The model under review builds one solid part; all positions refer to its coordinate system, in mm. A direction names the side the tool comes from. Give positions to 0.01 mm unless a question says otherwise; leave off trailing zeros. Loops run counter-clockwise (first coordinate to the right, second up) from the corner with the lowest first, then second, coordinate; pieces in that order, holes last. Notation, with made-up numbers: M 13,-29 L 63,-29 A28 ccw 63,-6 Z; hole C 12.25,41.25 d3. An arc over 180 degrees is marked long. Put each result on its own line as item: value. Start each with the question number.
from build123d import *

# Parameters (mm, degrees)
SKETCH1_W           = 30
SKETCH1_H           = 15
BOSS_EXTRUDE1_DEPTH = 3
SKETCH2_W           = 10
SKETCH2_H           = 15
BOSS_EXTRUDE2_DEPTH = 10
SKETCH3_R           = 2
CUT_EXTRUDE1_DEPTH  = 30
FILLET1_R           = 2


with BuildPart() as part:
    # Sketch1 → Boss-Extrude1 (new body)
    with BuildSketch(Plane(origin=(0, 0, 0), x_dir=(1, 0, 0), z_dir=(0, 1, 0))):
        with Locations((15, 7.5)):
            Rectangle(SKETCH1_W, SKETCH1_H)
    extrude(amount=BOSS_EXTRUDE1_DEPTH)

    # Sketch2 → Boss-Extrude2 (add)
    with BuildSketch(Plane(origin=(0, 3, 0), x_dir=(1, 0, 0), z_dir=(0, 1, 0))):
        with Locations((5, 7.5)):
            Rectangle(SKETCH2_W, SKETCH2_H)
        with Locations((25, 7.5)):
            Rectangle(SKETCH2_W, SKETCH2_H)
    extrude(amount=BOSS_EXTRUDE2_DEPTH)

    # Sketch3 → Cut-Extrude1 (cut)
    with BuildSketch(Plane.XZ):
        with Locations(Location((5, -7.5, 0), (0, 0, 270))):
            Circle(SKETCH3_R)
        with Locations(Location((25, -7.5, 0), (0, 0, 270))):
            Circle(SKETCH3_R)
    extrude(amount=-CUT_EXTRUDE1_DEPTH, mode=Mode.SUBTRACT)

    # Fillet1
    # the kernel refuses this fillet: 2 mm, written as the material it adds along each edge
    with BuildSketch(Plane(origin=(10, 3, -15), x_dir=(0, 1, 0), z_dir=(0, 0, 1)), Plane(origin=(20, 3, -15), x_dir=(-1, 0, 0), z_dir=(0, 0, 1))) as fillet1_piece_1:
        with BuildLine():
            CenterArc((FILLET1_R, -FILLET1_R), FILLET1_R, 90, 90)
            Line((0, -FILLET1_R), (0, 0))
            Line((0, 0), (FILLET1_R, 0))
        make_face()
    extrude(amount=15)
    # the kernel refuses this fillet: 2 mm, written as the material it takes off along each edge
    with BuildSketch(Plane(origin=(28, 2, -13), x_dir=(0, 0, -1), z_dir=(0, -1, 0))) as fillet1_2_piece_1_section:
        Polygon((0, 0), (FILLET1_R, 0), (FILLET1_R, FILLET1_R), (0, FILLET1_R), align=None)
    fillet1_2_piece_1 = extrude(amount=FILLET1_R, mode=Mode.PRIVATE)
    fillet1_2_piece_1 = fillet1_2_piece_1 - Plane(origin=(28, 2, -13), x_dir=(-0.7071067811865475, 0, 0.7071067811865475), z_dir=(0, -1, 0)) * Sphere(FILLET1_R, mode=Mode.PRIVATE)
    add(fillet1_2_piece_1, mode=Mode.SUBTRACT)
    with BuildSketch(Plane(origin=(2, 2, -13), x_dir=(0, 0, -1), z_dir=(0, -1, 0))) as fillet1_2_piece_2_section:
        Polygon((0, 0), (FILLET1_R, 0), (FILLET1_R, -FILLET1_R), (0, -FILLET1_R), align=None)
    fillet1_2_piece_2 = extrude(amount=FILLET1_R, mode=Mode.PRIVATE)
    fillet1_2_piece_2 = fillet1_2_piece_2 - Plane(origin=(2, 2, -13), x_dir=(0.7071067811865475, 0, 0.7071067811865475), z_dir=(0, -1, 0)) * Sphere(FILLET1_R, mode=Mode.PRIVATE)
    add(fillet1_2_piece_2, mode=Mode.SUBTRACT)
    with BuildSketch(Plane(origin=(28, 2, -2), x_dir=(0, 0, 1), z_dir=(0, -1, 0))) as fillet1_2_piece_3_section:
        Polygon((0, 0), (FILLET1_R, 0), (FILLET1_R, -FILLET1_R), (0, -FILLET1_R), align=None)
    fillet1_2_piece_3 = extrude(amount=FILLET1_R, mode=Mode.PRIVATE)
    fillet1_2_piece_3 = fillet1_2_piece_3 - Plane(origin=(28, 2, -2), x_dir=(-0.7071067811865475, 0, -0.7071067811865475), z_dir=(0, -1, 0)) * Sphere(FILLET1_R, mode=Mode.PRIVATE)
    add(fillet1_2_piece_3, mode=Mode.SUBTRACT)
    with BuildSketch(Plane(origin=(2, 2, -2), x_dir=(0, -1, 0), z_dir=(0, 0, 1))) as fillet1_2_piece_4_section:
        Polygon((0, 0), (FILLET1_R, 0), (FILLET1_R, -FILLET1_R), (0, -FILLET1_R), align=None)
    fillet1_2_piece_4 = extrude(amount=FILLET1_R, mode=Mode.PRIVATE)
    fillet1_2_piece_4 = fillet1_2_piece_4 - Plane(origin=(2, 2, -2), x_dir=(0.7071067811865475, 0.7071067811865475, 0), z_dir=(0, 0, 1)) * Sphere(FILLET1_R, mode=Mode.PRIVATE)
    add(fillet1_2_piece_4, mode=Mode.SUBTRACT)
    with BuildSketch(Plane(origin=(28, 0, -15), x_dir=(0, 0, 1), z_dir=(-1, 0, 0))) as fillet1_2_piece_5:
        with BuildLine():
            CenterArc((FILLET1_R, FILLET1_R), FILLET1_R, 180, 90)
            Line((0, FILLET1_R), (0, 0))
            Line((0, 0), (FILLET1_R, 0))
        make_face()
    extrude(amount=26, mode=Mode.SUBTRACT)
    with BuildSketch(Plane(origin=(30, 0, -2), x_dir=(0, 1, 0), z_dir=(0, 0, -1)), Plane(origin=(0, 0, -13), x_dir=(0, 1, 0), z_dir=(0, 0, 1))) as fillet1_2_piece_6:
        with BuildLine():
            CenterArc((FILLET1_R, -FILLET1_R), FILLET1_R, 90, 90)
            Line((0, -FILLET1_R), (0, 0))
            Line((0, 0), (FILLET1_R, 0))
        make_face()
    extrude(amount=11, mode=Mode.SUBTRACT)
    with BuildSketch(Plane(origin=(2, 0, 0), x_dir=(0, 1, 0), z_dir=(1, 0, 0))) as fillet1_2_piece_7:
        with BuildLine():
            CenterArc((FILLET1_R, -FILLET1_R), FILLET1_R, 90, 90)
            Line((0, -FILLET1_R), (0, 0))
            Line((0, 0), (FILLET1_R, 0))
        make_face()
    extrude(amount=26, mode=Mode.SUBTRACT)
    with BuildSketch(Plane(origin=(0, 18, -15), x_dir=(0, 0, 1), z_dir=(0, -1, 0)), Plane(origin=(30, 2, -15), x_dir=(0, 0, 1), z_dir=(0, 1, 0)), Plane(origin=(30, 2, 0), x_dir=(-1, 0, 0), z_dir=(0, 1, 0)), Plane(origin=(0, 18, 0), x_dir=(1, 0, 0), z_dir=(0, -1, 0))) as fillet1_2_piece_8:
        with BuildLine():
            CenterArc((FILLET1_R, -FILLET1_R), FILLET1_R, 90, 90)
            Line((0, -FILLET1_R), (0, 0))
            Line((0, 0), (FILLET1_R, 0))
        make_face()
    extrude(amount=16, mode=Mode.SUBTRACT)
    # the kernel refuses this fillet: 2 mm, written as the material it takes off along each edge
    with BuildSketch(Plane(origin=(12, 3, 0), x_dir=(0, -1, 0), z_dir=(1, 0, 0))) as fillet1_3_piece_1:
        with BuildLine():
            CenterArc((FILLET1_R, FILLET1_R), FILLET1_R, 180, 90)
            Line((0, FILLET1_R), (0, 0))
            Line((0, 0), (FILLET1_R, 0))
        make_face()
    extrude(amount=6, mode=Mode.SUBTRACT)
    with BuildSketch(Plane(origin=(10, 5, 0), x_dir=(-1, 0, 0), z_dir=(0, 1, 0)), Plane(origin=(10, 5, -15), x_dir=(0, 0, 1), z_dir=(0, 1, 0))) as fillet1_3_piece_2:
        with BuildLine():
            CenterArc((FILLET1_R, -FILLET1_R), FILLET1_R, 90, 90)
            Line((0, -FILLET1_R), (0, 0))
            Line((0, 0), (FILLET1_R, 0))
        make_face()
    extrude(amount=13, mode=Mode.SUBTRACT)
    with BuildSketch(Plane(origin=(18, 3, -15), x_dir=(0, 0, 1), z_dir=(-1, 0, 0))) as fillet1_3_piece_3:
        with BuildLine():
            CenterArc((FILLET1_R, -FILLET1_R), FILLET1_R, 90, 90)
            Line((0, -FILLET1_R), (0, 0))
            Line((0, 0), (FILLET1_R, 0))
        make_face()
    extrude(amount=6, mode=Mode.SUBTRACT)
    with BuildSketch(Plane(origin=(20, 5, -15), x_dir=(0, 0, 1), z_dir=(0, 1, 0)), Plane(origin=(20, 5, 0), x_dir=(1, 0, 0), z_dir=(0, 1, 0))) as fillet1_3_piece_4:
        with BuildLine():
            CenterArc((FILLET1_R, FILLET1_R), FILLET1_R, 180, 90)
            Line((0, FILLET1_R), (0, 0))
            Line((0, 0), (FILLET1_R, 0))
        make_face()
    extrude(amount=13, mode=Mode.SUBTRACT)
    with BuildSketch(Plane(origin=(18, 5, 0), x_dir=(0, -1, 0), z_dir=(-1, 0, 0))) as fillet1_3_piece_5:
        with BuildLine():
            CenterArc((2 + FILLET1_R, -FILLET1_R), FILLET1_R, 90, 90)
            Line((2, -FILLET1_R), (2, 0))
            Line((2, 0), (2 + FILLET1_R, 0))
        make_face()
    revolve(axis=Axis((18, 5, 0), (0, 0, 1)), revolution_arc=90, mode=Mode.SUBTRACT)
    with BuildSketch(Plane(origin=(18, 5, -15), x_dir=(0, -1, 0), z_dir=(-1, 0, 0))) as fillet1_3_piece_6:
        with BuildLine():
            CenterArc((2 + FILLET1_R, FILLET1_R), FILLET1_R, 180, 90)
            Line((2 + FILLET1_R, 0), (2, 0))
            Line((2, 0), (2, FILLET1_R))
        make_face()
    revolve(axis=Axis((18, 5, -15), (0, 0, 1)), revolution_arc=90, mode=Mode.SUBTRACT)
    with BuildSketch(Plane(origin=(12, 5, -15), x_dir=(-1, 0, 0), z_dir=(0, 1, 0))) as fillet1_3_piece_7:
        with BuildLine():
            CenterArc((2 + FILLET1_R, FILLET1_R), FILLET1_R, 180, 90)
            Line((2 + FILLET1_R, 0), (2, 0))
            Line((2, 0), (2, FILLET1_R))
        make_face()
    revolve(axis=Axis((12, 5, -15), (0, 0, 1)), revolution_arc=90, mode=Mode.SUBTRACT)
    with BuildSketch(Plane(origin=(12, 5, 0), x_dir=(-1, 0, 0), z_dir=(0, 1, 0))) as fillet1_3_piece_8:
        with BuildLine():
            CenterArc((2 + FILLET1_R, -FILLET1_R), FILLET1_R, 90, 90)
            Line((2, -FILLET1_R), (2, 0))
            Line((2, 0), (2 + FILLET1_R, 0))
        make_face()
    revolve(axis=Axis((12, 5, 0), (0, 0, 1)), revolution_arc=90, mode=Mode.SUBTRACT)


solid = part.part
(1) For faces 5 (the flat face through (15, 3, -8)), 6 (the cylindrical face through (9.4, 8.94, -0.57)), 7 (the flat face through (3.8, 13, -9.3)), 8 (the cylindrical face through (15, 2.6, -14.2)), list the 3-axis set-ups (+Z, -Z, +X, -X, +Y, -Y) from which the entire face can be reached by the end or side of a thin tool; tool diameter is ignored.
(2) Insertion check: pin 1 (6.5 mm diameter, centred on x = 13.5, z = -8.5, fed in from +Y); pin 2 (4 mm diameter, centred on x = 11.5, y = 7, fed in from -Z). Each pin has a flat end and moves straight along its axis. Give the tip position at first contact, or say it passes through.
(3) Draft analysis for pull direction Z (two halves, no side actions). For faces 1 (the cylindrical face through (23.8, 6.4, -5.9)), 2 (the cylindrical face through (9.43, 8.94, -14.4)), 3 (the cylindrical face through (14.82, 0.6, -0.57)), 4 (the cylindrical face through (10.57, 3.6, -7.58)), state which applies: +Z half, -Z half, draft (parallel to the pull), parting line (faces both ways), or undercut.
(4) We need section D-D, the plane z = -10.5. Write out the cut boundary in (x, y).
(5) We need section B-B, the plane x = 25. Write out the cut boundary in (y, z), plus the area to 3 significant figures.
(6) We need section A-A, the plane y = 8.5. Write out the cut boundary in (x, z), plus the area to 3 significant figures.
(7) We need section C-C, the plane z = -7.5. Write out the cut boundary in (x, y), plus the area to 3 significant figures.
(8) To check wall thickness, follow L1, parallel to X at y = 7.5, z = -11; L2, parallel to X at y = 6.5, z = -6.75; L3, parallel to Z at x = 23.5, y = 4.25. State the ranges of each line that lie inside material, in increasing order. Write a range as [from, to].
Check sheet entries:
1. face 5: +Z, -Z, +Y
1. face 6: +Z, +Y
1. face 7: +Z, -Z, +X, -X, +Y
1. face 8: -Z, +Y
2. pin 1: stops at y = 4.03
2. pin 2: stops at z = -14.32
3. face 1: undercut
3. face 2: -Z half
3. face 3: +Z half
3. face 4: draft
4. outline: M 0,2 A2 ccw 2,0 L 28,0 A2 ccw 30,2 L 30,13 L 20,13 L 20,5 A2 cw 18,3 L 12,3 A2 cw 10,5 L 10,13 L 0,13 Z
5. outline: M 0,-13 A2 ccw 2,-15 L 13,-15 L 13,-9.5 L 0,-9.5 Z; M 0,-5.5 L 13,-5.5 L 13,0 L 2,0 A2 ccw 0,-2 Z
5. area: 141 mm²
6. outline: M 0,-13 A2 ccw 2,-15 L 8,-15 A2 ccw 10,-13 L 10,-2 A2 ccw 8,0 L 2,0 A2 ccw 0,-2 Z; M 20,-13 A2 ccw 22,-15 L 28,-15 A2 ccw 30,-13 L 30,-2 A2 ccw 28,0 L 22,0 A2 ccw 20,-2 Z; hole C 5,-7.5 d4; hole C 25,-7.5 d4
6. area: 268 mm²
7. outline: M 0,2 A2 ccw 2,0 L 3,0 L 3,13 L 0,13 Z; M 7,0 L 23,0 L 23,13 L 20,13 L 20,5 A2 cw 18,3 L 12,3 A2 cw 10,5 L 10,13 L 7,13 Z; M 27,0 L 28,0 A2 ccw 30,2 L 30,13 L 27,13 Z
7. area: 186 mm²
8. L1: x = [0, 10], [20, 30]
8. L2: x = [0, 3.15], [6.85, 10], [20, 23.15], [26.85, 30]
8. L3: z = [-15, -8.82], [-6.18, 0]
